The model under review builds one solid part; all positions refer to its coordinate system, in mm. A direction names the side the tool comes from. Coordinates: 2 decimals unless noted, no trailing zeros. Order: outer loops, then holes, each group sorted by start corner. A loop starts at its lowest first (then second) coordinate and runs counter-clockwise, first axis right, second up. Notation, with made-up numbers: (-23.5, 25) -> (7.5, 25) arc R20 ccw to (7.5, 32) -> close; hole circle Ø11 at (72.5, 67). An arc over 180 degrees is marked (long way). Use one line per item in the form item = value. Start each with the question number.
(1) Mouldability with a two-part tool opening along X and no side actions: class faces 3 (the flat face through (0, -3, 0)), 4 (the cylindrical face through (1.08, -4.88, 7.69)), 5 (the cylindrical face through (0.325, 10.464, 1.774)) as +X half, -X half, draft (parallel to the pull), parting line (faces both ways), or undercut.
(2) Insertion check: pin 1 Ø2 at (y, z) = (4.5, 4) entering from +X; pin 2 Ø2.5 at (x, y) = (9, 0) entering from -Z; pin 3 Ø1 at (x, z) = (5, 8.5) entering from +Y; pin 4 Ø4 at (y, z) = (-7, 2) entering from -X. Each pin has a flat end and moves straight along its axis. Give the tip position at first contact, or say it passes through.
(3) Take a section at A-A (x = 0). State the section outline as (y, z) points.
(4) Take a section at C-C (y = -8.5). State the section outline as (x, z) points, then the cut area to 3 significant figures.
(5) Take a section at D-D (z = 2). State the section outline as (x, y) points, then the cut area to 3 significant figures.
(6) Wall thickness on line 1 along Y through (x, z) = (0, 1); line 2 along Y through (x, z) = (0, 8.25); line 3 along Z through (x, y) = (0.75, -7): over which ranges is each line inside the solid? List them lowest first.
(7) Take a section at B-B (x = -9). State the section outline as (y, z) points.
(8) For faces 1 (the cylindrical face through (10.5, -0.07, 1.77)), 2 (the flat face through (-0.2, -5.4, 3.5)), list the 3-axis set-ups (+Z, -Z, +X, -X, +Y, -Y) from which the entire face can be reached by the end or side of a thin tool; tool diameter is ignored.
Autodesk Fusion 360 part; units mm, degrees
sketch "スケッチ1" plane through (0, 0, 0) normal (0, 0, 1) x (1, 0, 0)
  circle A0 centre (0, 0) radius 12.5
  dimension "d1" = 25
extrude "押し出し1" add sketch "スケッチ1" along normal blind 3.5
sketch "スケッチ2" plane through (0, 0, 3.5) normal (0, 0, 1) x (-1, 0, 0)
  circle A0 centre (0, 0) radius 12.5
  circle A1 centre (0, 0) radius 5
  dimension "d4" = 10
extrude "押し出し2" add sketch "スケッチ2" along normal blind 8.5 contours A1
sketch "スケッチ3" plane through (0, 0, 12) normal (0, 0, 1) x (-1, 0, 0)
  circle A0 centre (0, 0) radius 5
  circle A1 centre (0, 0) radius 2.5
  dimension "d7" = 5
extrude "押し出し3" cut sketch "スケッチ3" against normal blind 12 contours A1
sketch "スケッチ4" plane through (0, 0, 3.5) normal (0, 0, 1) x (-1, 0, 0)
  circle A0 centre (0, 0) radius 5
  circle A1 centre (0, 0) radius 12.5
  line L0 (12.5, 0) -> (-12.5, 0)
  line L1 (0, 0) -> (-9, 0)
  line L2 (0, 0) -> (9, 0)
  circle A2 centre (-9, 0) radius 1.5
  circle A3 centre (0, -9) radius 1.5
  circle A4 centre (9, 0) radius 1.5
  circle A5 centre (0, 9) radius 1.5
  dimension "d10" = 25
  dimension "d11" = 9
  dimension "d12" = 9
  dimension "d13" = 3
  dimension "d15" = 360
extrude "押し出し4" cut sketch "スケッチ4" against normal blind 3.5 contours L0 L2 A4 | L0 L2 A4 | L0 L1 A2 | L0 L1 A2 | A3 | A5
sketch "スケッチ5" plane through (0, 0, 3.5) normal (0, 0, 1) x (-1, 0, 0)
  circle A0 centre (0, 9) radius 1.5
  circle A1 centre (9, 0) radius 1.5
  circle A2 centre (-9, 0) radius 1.5
  circle A3 centre (0, -9) radius 1.5
  circle A4 centre (0, 0) radius 5
  circle A5 centre (0, 0) radius 12.5
Findings:
q1.face_3 = draft
q1.face_4 = parting line
q1.face_5 = undercut
q2.pin_1 = 11.96
q2.pin_2 = through
q2.pin_3 = 2.18
q2.pin_4 = -11.46
q3.outline = (-12.5, 0) -> (-10.5, 0) -> (-10.5, 3.5) -> (-12.5, 3.5) -> close; (-7.5, 0) -> (-2.5, 0) -> (-2.5, 12) -> (-5, 12) -> (-5, 3.5) -> (-7.5, 3.5) -> close; (2.5, 0) -> (7.5, 0) -> (7.5, 3.5) -> (5, 3.5) -> (5, 12) -> (2.5, 12) -> close; (10.5, 0) -> (12.5, 0) -> (12.5, 3.5) -> (10.5, 3.5) -> close
q4.outline = (-9.17, 0) -> (-1.41, 0) -> (-1.41, 3.5) -> (-9.17, 3.5) -> close; (1.41, 0) -> (9.17, 0) -> (9.17, 3.5) -> (1.41, 3.5) -> close
q4.area = 54.3 mm²
q5.outline = circle Ø25 at (0, 0); hole circle Ø3 at (-9, 0); hole circle Ø5 at (0, 0); hole circle Ø3 at (0, -9); hole circle Ø3 at (0, 9); hole circle Ø3 at (9, 0)
q5.area = 443 mm²
q6.line_1 = -12.5 to -10.5, -7.5 to -2.5, 2.5 to 7.5, 10.5 to 12.5
q6.line_2 = -5 to -2.5, 2.5 to 5
q6.line_3 = 0 to 3.5
q7.outline = (-8.67, 0) -> (-1.5, 0) -> (-1.5, 3.5) -> (-8.67, 3.5) -> close; (1.5, 0) -> (8.67, 0) -> (8.67, 3.5) -> (1.5, 3.5) -> close
q8.face_1 = +Z, -Z
q8.face_2 = +Z
